Check sheet for the modelled part. Datum: model origin and axes. Units: mm. Face numbers are marked on the shaded views. A direction names the side the tool comes from. Coordinates: 2 decimals unless noted, no trailing zeros. Loops run counter-clockwise (first coordinate to the right, second up) from the corner with the lowest first, then second, coordinate; pieces in that order, holes last. Notation, with made-up numbers: (7.5, 88) - (43.5, 88) arc R21 cw to (43.5, 126) - close; hole circle Ø7 at (63, 67). An arc over 180 degrees is marked (long way). Use a Markdown table: item, result. Add a question column.
1) Sectioned sample at A-A, the plane z = 0. Enter the section's corners in (x, y) (3 decimals).
2) Thickness scan on line 1 (Z direction, x = 0, y = 4.5) (3 decimals); line 2 (Z direction, x = -35.5, y = -6); line 3 (X direction, y = -17, z = 35). Record the ranges inside material, lowest first.
3) Sectioned sample at C-C, the plane y = 4.5. Enter the section's corners in (x, z) (3 decimals).
4) Draft check along Z on the marked faces 1, 2, 3 and 4. Enter one of: pulls with the +Z half, pulls with the -Z half, needs draft (parallel to the pull), parting line crosses it, or undercut.
5) Sectioned sample at B-B, the plane x = 0. Enter the section's corners in (y, z) (3 decimals).
6) Sectioned sample at D-D, the plane z = -59.5. Enter the section's corners in (x, y).
7) Tool access check on the marked faces 5, 6 and 7. Record the directions out of +Z, -Z, +X, -X, +Y, -Y that give a thin tool (end or side, any length) a straight path to the whole face; none if there is none.
8) Go/stop test with flat-tipped pins: P1, Ø1.5, axis at y = -20, z = 34.5, coming from the -X side; P2, Ø6, axis at y = -1, z = 37.5, coming from the +X side; P3, Ø1.5, axis at y = -16.5, z = -4, coming from the -X side; P4, Ø23, axis at x = 0, z = 0, coming from the -Y side. Record where each tip stops, or that it passes through.
Autodesk Inventor part; units mm, degrees
ref_plane "YZ Plane" through (0, 0, 0) normal (1, 0, 0) x (0, 1, 0)
ref_plane "XZ Plane" through (0, 0, 0) normal (0, 1, 0) x (-1, 0, 0)
ref_plane "XY Plane" through (0, 0, 0) normal (0, 0, 1) x (1, 0, 0)
sketch "Sketch1" plane through (0, 0, 0) normal (0, 1, 0) x (-1, 0, 0)
  arc A0 (38.1, -38.2321) -> (-38.1, -38.2321) centre (0, 0) ccw
  line L0 (0, 0) -> (0, -72.7817) construction
  line L1 (-38.1, -38.2321) -> (-38.1, -69.85)
  line L2 (-38.1, -69.85) -> (0, -69.85)
  line L3 (0, -69.85) -> (38.1, -69.85)
  line L4 (38.1, -69.85) -> (38.1, -38.2321)
  dimension "d0" = 107.95
  dimension "d6" = 69.85
  dimension "d7" = 38.1
extrude "Extrusion1" add sketch "Sketch1" along normal blind 6.35
sketch "Sketch3" plane through (0, 0, 0) normal (0, -1, 0) x (1, 0, 0)
  arc A0 (38.1, -38.2321) -> (-38.1, -38.2321) centre (0, 0) ccw
  line L0 (38.1, -38.2321) -> (38.1, -69.85)
  line L1 (38.1, -69.85) -> (-38.1, -69.85)
  line L2 (-38.1, -69.85) -> (-38.1, -38.2321)
  arc A1 (38.1, -38.2321) -> (-38.1, -38.2321) centre (0, 0) ccw
  line L3 (38.1, -38.2321) -> (38.1, -69.85)
  line L4 (38.1, -38.2321) -> (38.1, -69.85)
  line L5 (38.1, -69.85) -> (-38.1, -69.85)
  line L6 (-38.1, -69.85) -> (-38.1, -38.2321)
  line L7 (-38.1, -69.85) -> (-38.1, -38.2321)
  arc A2 (44.45, -40.7836) -> (-44.45, -40.7836) centre (0, 0) ccw
  line L8 (44.45, -40.7836) -> (44.45, -76.2)
  line L9 (44.45, -76.2) -> (-44.45, -76.2)
  line L10 (-44.45, -76.2) -> (-44.45, -40.7836)
  dimension "d8" = 6.35
  dimension "d9" = 6.35
  dimension "d10" = 6.35
  dimension "d11" = 6.35
extrude "Extrusion3" add sketch "Sketch3" along normal blind 25.4
extrude "Extrusion4" add sketch "Sketch3" against normal blind 6.35
sketch "Sketch4" plane through (44.45, -25.4, -40.7836) normal (1, 0, 0) x (0, 0, -1)
  line L0 (20.7014, 17.1105) -> (20.7014, 11.6112)
  line L1 (10.9224, 11.4645) -> (10.9224, 17.1105)
  line L2 (15.6849, 8.7149) -> (10.9224, 11.4645)
  line L3 (20.7014, 11.6112) -> (15.6849, 8.7149)
  line L4 (15.8119, 19.9334) -> (20.7014, 17.1105)
  line L5 (10.9224, 17.1105) -> (15.8119, 19.9334)
  line L6 (10.9224, 17.1105) -> (20.7014, 11.6112) construction
  line L7 (10.9224, 11.4645) -> (20.7014, 17.1105) construction
  circle A0 centre (15.8119, 14.2875) radius 7.9375
  line L8 (20.5744, 17.0371) -> (20.5744, 11.5379)
  line L9 (20.5744, 11.5379) -> (15.8119, 8.7882)
  line L10 (15.8119, 8.7882) -> (11.0494, 11.5379)
  line L11 (11.0494, 11.5379) -> (11.0494, 17.0371)
  line L12 (11.0494, 17.0371) -> (15.8119, 19.7868)
  line L13 (15.8119, 19.7868) -> (20.5744, 17.0371)
  point P0 (-40.7836, 25.4)
  dimension "d20" = 15.875
  dimension "d21" = 9.525
extrude "Extrusion6" cut sketch "Sketch4" against normal up to surface (6.35 mm away) contours L0 L3 L8 L13 L12 L11 L10 L2 L1 L5 L4 | L3 L10 L11 L12 L13 L8 | A0
mirror "Mirror1" about plane through (0, 0, 0) normal (1, 0, 0) of "Extrusion6"
sketch "Sketch5" plane through (0, 6.35, 0) normal (0, 1, 0) x (1, 0, 0)
  circle A0 centre (0, 0) radius 12.7
  dimension "d24" = 25.4
extrude "Extrusion7" cut sketch "Sketch5" against normal through all
equation "\"d0\" = exteriorDiameter"
equation "\"exteriorDiameter\" = 107.95"
properties part number "baseSupport"
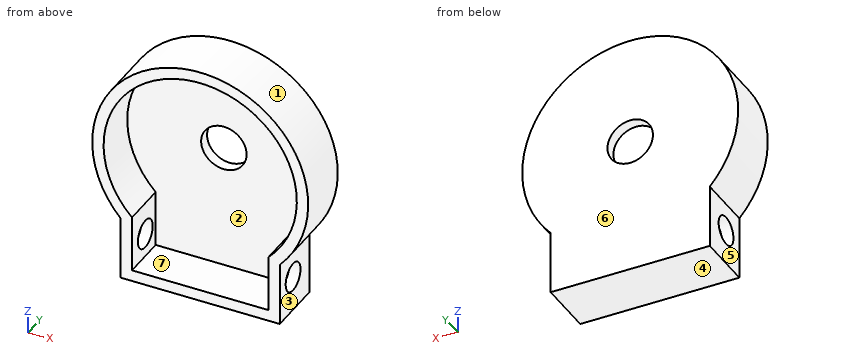
Solved:
| question | item | result |
|---|---|---|
| 1 | outline | (-60.325, -25.4) - (-53.975, -25.4) - (-53.975, 0) - (-12.7, 0) - (-12.7, 6.35) - (-60.325, 6.35) - close; (12.7, 0) - (53.975, 0) - (53.975, -25.4) - (60.325, -25.4) - (60.325, 6.35) - (12.7, 6.35) - close |
| 2 | line 1 | z = -76.2 to -12.7, 12.7 to 60.325 |
| 2 | line 2 | z = -76.2 to -69.85, 40.66 to 48.77 |
| 2 | line 3 | x = -49.13 to -41.09, 41.09 to 49.13 |
| 3 | outline | (-44.45, -76.2) - (44.45, -76.2) - (44.45, -40.784) arc R60.325 ccw (long way) to (-44.45, -40.784) - close; hole circle Ø25.4 at (0, 0) |
| 4 | face 1 | parting line crosses it |
| 4 | face 2 | undercut |
| 4 | face 3 | needs draft |
| 4 | face 4 | pulls with the -Z half |
| 5 | outline | (-25.4, -76.2) - (6.35, -76.2) - (6.35, -12.7) - (0, -12.7) - (0, -69.85) - (-25.4, -69.85) - close; (-25.4, 53.975) - (0, 53.975) - (0, 12.7) - (6.35, 12.7) - (6.35, 60.325) - (-25.4, 60.325) - close |
| 6 | outline | (-44.45, -25.4) - (-38.1, -25.4) - (-38.1, -18.5) - (-44.45, -18.5) - close; (-44.45, -3.73) - (-38.1, -3.73) - (-38.1, 0) - (38.1, 0) - (38.1, -3.73) - (44.45, -3.73) - (44.45, 6.35) - (-44.45, 6.35) - close; (38.1, -25.4) - (44.45, -25.4) - (44.45, -18.5) - (38.1, -18.5) - close |
| 7 | face 5 | -Z, -X, +Y, -Y |
| 7 | face 6 | +Z, -Z, +X, -X, +Y |
| 7 | face 7 | -Y |
| 8 | P1 | stops at x = -50 |
| 8 | P2 | stops at x = 49.49 |
| 8 | P3 | stops at x = -60.24 |
| 8 | P4 | passes through |
